Work out the finished part from the listing and answer in its coordinate system (mm). A direction names the side the tool comes from. Round coordinates to 2 decimals unless told otherwise and drop trailing zeros. Order: outer loops, then holes, each group sorted by start corner. A loop starts at its lowest first (then second) coordinate and runs counter-clockwise, first axis right, second up. Notation, with made-up numbers: (-15.5, -1) -> (34.5, -1) arc R10 cw to (34.5, 3) -> close; hole circle Ø9 at (-0.5, 19.25). An arc over 180 degrees is marked (long way). Use a Markdown table: item, result. Add a question column.
Item 1: For a pull along X with two mould halves and no side action, classify faces 3 (the flat face through (1, 1, 0)), 4 (the cylindrical face through (-2.43, 3.04, -2.4)), 5 (the flat face through (3, 3, 0)) as +X half, -X half, draft (parallel to the pull), parting line (faces both ways), or undercut.
Item 2: A cutting plane is placed at C-C, the plane z = 0. Determine the outline of the cut face in (x, y).
Item 3: A tool of negligible diameter and unlimited length cuts with its end or side. For faces 1 (the flat face through (-3, 3, 0)), 2 (the flat face through (-1, 1, 0)), from which of +Z, -Z, +X, -X, +Y, -Y can it reach the whole face along a straight path? Write none if from no direction.
Item 4: A cutting plane is placed at B-B, the plane x = 0.75. Determine the outline of the cut face in (y, z).
Item 5: Find the intervals of material crossed by L1, parallel to Z at x = 0.75, y = 2.2; L2, parallel to Z at x = -1.5, y = 3.5, in increasing order. Write a range as [from, to].
Item 6: A cutting plane is placed at D-D, the plane y = 4.8. Determine the outline of the cut face in (x, z).
Item 7: A cutting plane is placed at A-A, the plane y = 0.9. Determine the outline of the cut face in (x, z).
from build123d import *

# Parameters (mm, degrees)
SKETCH1_W           = 6
SKETCH1_H           = 6
BOSS_EXTRUDE1_DEPTH = 6
SKETCH2_W           = 2
SKETCH2_H           = 2
CUT_EXTRUDE1_DEPTH  = 2.5
FILLET1_R           = 2
CHAMFER1_SIZE       = 0.3
CHAMFER1_SIZE2      = 0.519615242


with BuildPart() as part:
    # Sketch1 → Boss-Extrude1 (new body)
    with BuildSketch(Plane(origin=(0, 0, 0), x_dir=(1, 0, 0), z_dir=(0, 1, 0))):
        Rectangle(SKETCH1_W, SKETCH1_H)
    extrude(amount=BOSS_EXTRUDE1_DEPTH)

    # Sketch2 → Cut-Extrude1 (cut)
    with BuildSketch(Plane.XZ):
        Rectangle(SKETCH2_W, SKETCH2_H)
    extrude(amount=-CUT_EXTRUDE1_DEPTH, mode=Mode.SUBTRACT)

    # Fillet1
    fillet1_edges = [part.edges().sort_by_distance(p)[0] for p in [
        (-3, 3, -3),
        (3, 3, -3),
        (3, 3, 3),
        (-3, 3, 3),
    ]]
    fillet(fillet1_edges, radius=FILLET1_R)

    # Chamfer1
    chamfer1_edges = [part.edges().sort_by_distance(p)[0] for p in [
        (-1, 0, 0),
        (0, 0, -1),
        (1, 0, 0),
        (0, 0, 1),
    ]]
    chamfer1_side = [part.faces().sort_by_distance(p)[0] for p in [
        (0, 0, 2.915147186),
    ]]
    chamfer(chamfer1_edges, length=CHAMFER1_SIZE, length2=CHAMFER1_SIZE2, reference=chamfer1_side[0])


solid = part.part
Reported:
| question | item | result |
|---|---|---|
| 1 | face 3 | undercut |
| 1 | face 4 | -X half |
| 1 | face 5 | +X half |
| 2 | outline | (-3, 0) -> (-1.3, 0) -> (-1, 0.52) -> (-1, 2.5) -> (1, 2.5) -> (1, 0.52) -> (1.3, 0) -> (3, 0) -> (3, 6) -> (-3, 6) -> close |
| 3 | face 1 | +Z, -Z, -X, +Y, -Y |
| 3 | face 2 | -Y |
| 4 | outline | (0, -3) -> (6, -3) -> (6, 3) -> (0, 3) -> (0, 1.3) -> (0.52, 1) -> (2.5, 1) -> (2.5, -1) -> (0.52, -1) -> (0, -1.3) -> close |
| 5 | L1 | [-3, -1], [1, 3] |
| 5 | L2 | [-2.94, 2.94] |
| 6 | outline | (-3, -1) arc R2 ccw to (-1, -3) -> (1, -3) arc R2 ccw to (3, -1) -> (3, 1) arc R2 ccw to (1, 3) -> (-1, 3) arc R2 ccw to (-3, 1) -> close |
| 7 | outline | (-3, -1) arc R2 ccw to (-1, -3) -> (1, -3) arc R2 ccw to (3, -1) -> (3, 1) arc R2 ccw to (1, 3) -> (-1, 3) arc R2 ccw to (-3, 1) -> close; hole (-1, -1) -> (1, -1) -> (1, 1) -> (-1, 1) -> close |
